```python
from build123d import *

# Parameters (mm, degrees)
F0_R     = 23.00605
F0_R_2   = 19.431
F1_DEPTH = 77.47
F2_SIZE  = 2.54
F0_R_3   = 27.9781
F3_DEPTH = 1.5875


with BuildPart() as f1:
    # F0 (on Front) → F1 (new body, symmetric)
    with BuildSketch(Plane.XZ):
        Circle(F0_R)
        Circle(F0_R_2, mode=Mode.SUBTRACT)
    extrude(amount=F1_DEPTH, both=True)

    # F2
    f2_edges = [f1.edges().sort_by_distance(p)[0] for p in [
        (-23.00605, -77.47, 0),
        (-23.00605, 77.47, 0),
    ]]
    chamfer(f2_edges, length=F2_SIZE)

    # F0 (on Front) → F3 (join, symmetric)
    with BuildSketch(Plane.XZ):
        Circle(F0_R_3)
        Circle(F0_R, mode=Mode.SUBTRACT)
    extrude(amount=F3_DEPTH, both=True)


solid = f1.part
```
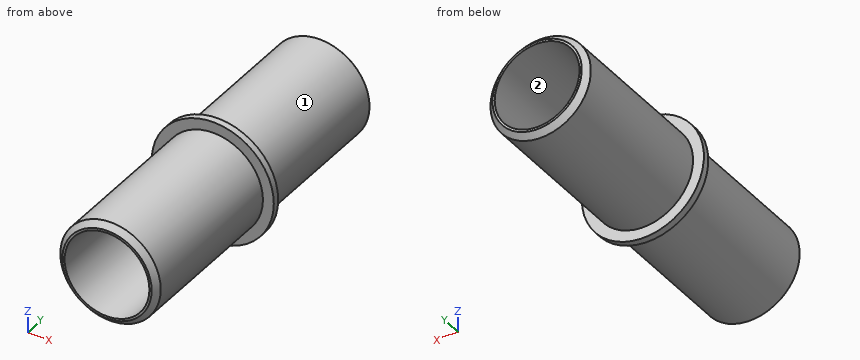
Build history of the part. All positions in model axes, mm. Face numbers are marked on the shaded views. Round coordinates to 2 decimals unless told otherwise and drop trailing zeros. Order: outer loops, then holes, each group sorted by start corner. A loop starts at its lowest first (then second) coordinate and runs counter-clockwise, first axis right, second up. Notation, with made-up numbers: (70.25, -15.75) - (129.25, -15.75) arc R8 cw to (129.25, -10.75) - close; hole circle Ø1 at (0.25, 61). An arc over 180 degrees is marked (long way). Use a Markdown table: item, result.
1) Saw through at D-D on y = 0. Write the cut outline in (x, z).
Recorded:
| item | result |
|---|---|
| outline | circle Ø55.96 at (0, 0); hole circle Ø38.86 at (0, 0) |
2) Wall check: L1, parallel to Z at x = -0.5, y = 70; L2, parallel to X at y = 33.5, z = -1; L3, parallel to X at y = 46.5, z = -4. Give the ranges that are in metal, low to high.
Recorded:
| item | result |
|---|---|
| L1 | z = -23 to -19.42, 19.42 to 23 |
| L2 | x = -22.98 to -19.41, 19.41 to 22.98 |
| L3 | x = -22.66 to -19.01, 19.01 to 22.66 |
3) Saw through at A-A on z = 0. Write the cut outline in (x, y), and give its area (3 significant figures).
Recorded:
| item | result |
|---|---|
| outline | (-27.98, -1.59) - (-23.01, -1.59) - (-23.01, -74.93) - (-20.47, -77.47) - (-19.43, -77.47) - (-19.43, 77.47) - (-20.47, 77.47) - (-23.01, 74.93) - (-23.01, 1.59) - (-27.98, 1.59) - close; (19.43, -77.47) - (20.47, -77.47) - (23.01, -74.93) - (23.01, -1.59) - (27.98, -1.59) - (27.98, 1.59) - (23.01, 1.59) - (23.01, 74.93) - (20.47, 77.47) - (19.43, 77.47) - close |
| area | 1,130 mm² |
4) Saw through at B-B on x = 0. Write the cut outline in (y, z), and give its area (3 significant figures).
Recorded:
| item | result |
|---|---|
| outline | (-77.47, -20.47) - (-74.93, -23.01) - (-1.59, -23.01) - (-1.59, -27.98) - (1.59, -27.98) - (1.59, -23.01) - (74.93, -23.01) - (77.47, -20.47) - (77.47, -19.43) - (-77.47, -19.43) - close; (-77.47, 19.43) - (77.47, 19.43) - (77.47, 20.47) - (74.93, 23.01) - (1.59, 23.01) - (1.59, 27.98) - (-1.59, 27.98) - (-1.59, 23.01) - (-74.93, 23.01) - (-77.47, 20.47) - close |
| area | 1,130 mm² |
5) Flat gauge pins, fed straight in: pin 1 Ø1 at (x, y) = (1.5, -24) entering from -Z; pin 2 Ø4 at (x, y) = (-16.5, 32) entering from -Z; pin 3 Ø8 at (x, y) = (-10.5, -8) entering from +Z; pin 4 Ø4 at (x, z) = (17.5, -5.5) entering from +Y. Where does each tip first touch, or does it go through?
Recorded:
| item | result |
|---|---|
| pin 1 | stops at z = -22.98 |
| pin 2 | stops at z = -17.86 |
| pin 3 | stops at z = 22.07 |
| pin 4 | stops at y = 77.47 |
6) Saw through at C-C on y = -25. Write the cut outline in (x, z), and give its area (3 significant figures).
Recorded:
| item | result |
|---|---|
| outline | circle Ø46.01 at (0, 0); hole circle Ø38.86 at (0, 0) |
| area | 477 mm² |
7) Pull direction X, two halves, no side cores. Call the marked faces 1 and 2: pulls with the +X half, pulls with the -X half, needs draft (parallel to the pull), parting line crosses it, or undercut.
Recorded:
| item | result |
|---|---|
| face 1 | parting line crosses it |
| face 2 | undercut |
